Check sheet for the drawn part. Datum: minimum x, y, z corner. Units: mm. A direction names the side the tool comes from. Round coordinates to 2 decimals unless told otherwise and drop trailing zeros. Write each loop counter-clockwise with the first axis right and the second up, starting at its lowest first coordinate (ties: lowest second). Pieces come first, ordered by that corner, then holes. Notation, with made-up numbers: M 73,-25.5 L 113,-25.5 A20 ccw 113,-7.5 Z; hole C 27,27 d7. An arc over 180 degrees is marked long. One line per item, written item: value. Start each with the question number.
Item 1: Section check B-B, the plane x = 27.4. Record the cut outline in (y, z), then the cut area to 3 significant figures.
Item 2: Section check A-A, the plane y = 22. Record the cut outline in (x, z), then the cut area to 3 significant figures.
Item 3: Draft check along X on the marked faces 1, 2 and 3. Enter one of: +X half, -X half, draft (parallel to the pull), parting line (faces both ways), or undercut.
Item 4: Tool access check on the marked faces 4 and 5. Record the directions out of +Z, -Z, +X, -X, +Y, -Y that give a thin tool (end or side, any length) a straight path to the whole face; none if there is none.
Item 5: Section check D-D, the plane x = 10.5. Record the cut outline in (y, z).
Item 6: Section check C-C, the plane z = 5.5. Record the cut outline in (x, y).
Item 7: Gauge pin test, flat ends, axial feed: pin 1 (0.9 mm diameter, centred on x = 2.5, z = 2.5, fed in from -Y); pin 2 (1.8 mm diameter, centred on x = 14.5, z = 2, fed in from -Y); pin 3 (4 mm diameter, centred on x = 10, y = 13.5, fed in from +Z); pin 4 (6 mm diameter, centred on x = 25, y = 18, fed in from -Z). Record the tip position at first contact, or that the pin passes through.
Item 8: Thickness scan on probe 1 along X at (y, z) = (20.5, 1.1); probe 2 along Z at (x, y) = (27.4, 7); probe 3 along X at (y, z) = (3, 3.75). Record the ranges inside material, lowest first. Write a range as from..to.
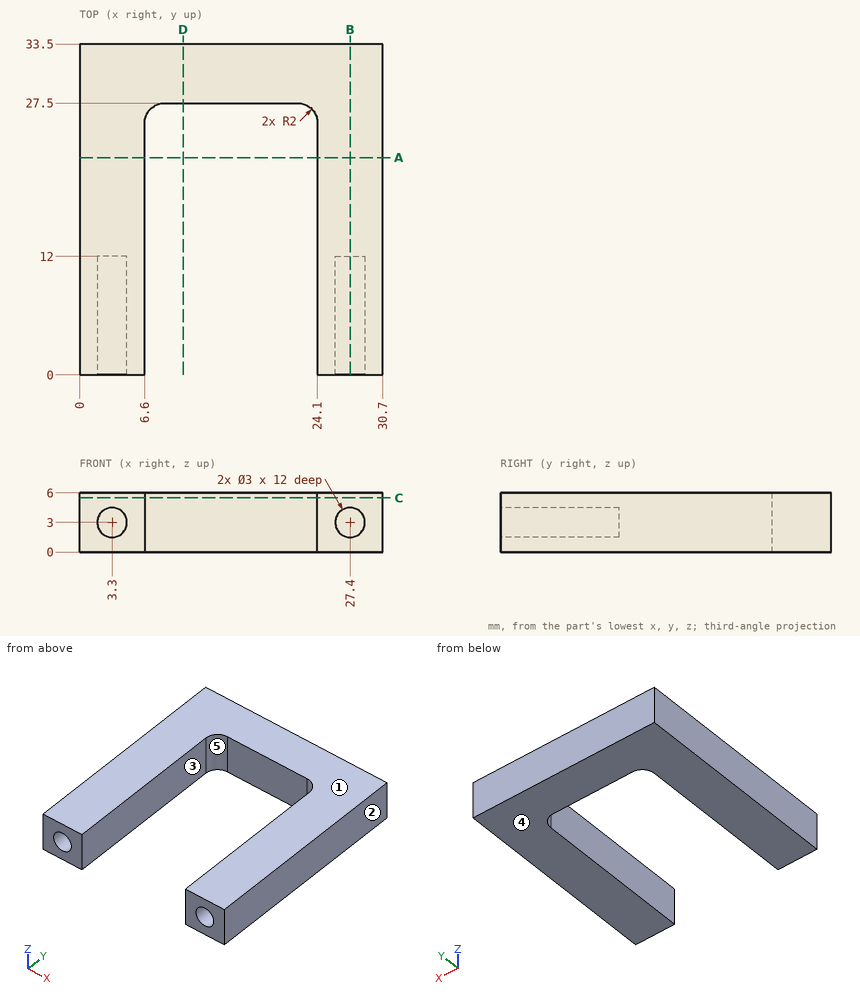
Response values:
1. outline: M 0,0 L 33.5,0 L 33.5,6 L 0,6 L 0,4.5 L 12,4.5 L 12,1.5 L 0,1.5 Z
1. area: 165 mm2
2. outline: M 0,0 L 6.6,0 L 6.6,6 L 0,6 Z; M 24.1,0 L 30.7,0 L 30.7,6 L 24.1,6 Z
2. area: 79.2 mm2
3. face 1: draft
3. face 2: +X half
3. face 3: undercut
4. face 4: -Z, +X, -X, +Y, -Y
4. face 5: +Z, -Z, -Y
5. outline: M 27.5,0 L 33.5,0 L 33.5,6 L 27.5,6 Z
6. outline: M 0,0 L 6.6,0 L 6.6,25.5 A2 cw 8.6,27.5 L 22.1,27.5 A2 cw 24.1,25.5 L 24.1,0 L 30.7,0 L 30.7,33.5 L 0,33.5 Z
7. pin 1: stops at y = 12
7. pin 2: stops at y = 27.5
7. pin 3: passes through
7. pin 4: stops at z = 0
8. probe 1: x = 0..6.6, 24.1..30.7
8. probe 2: z = 0..1.5, 4.5..6
8. probe 3: x = 0..2, 4.6..6.6, 24.1..26.1, 28.7..30.7
